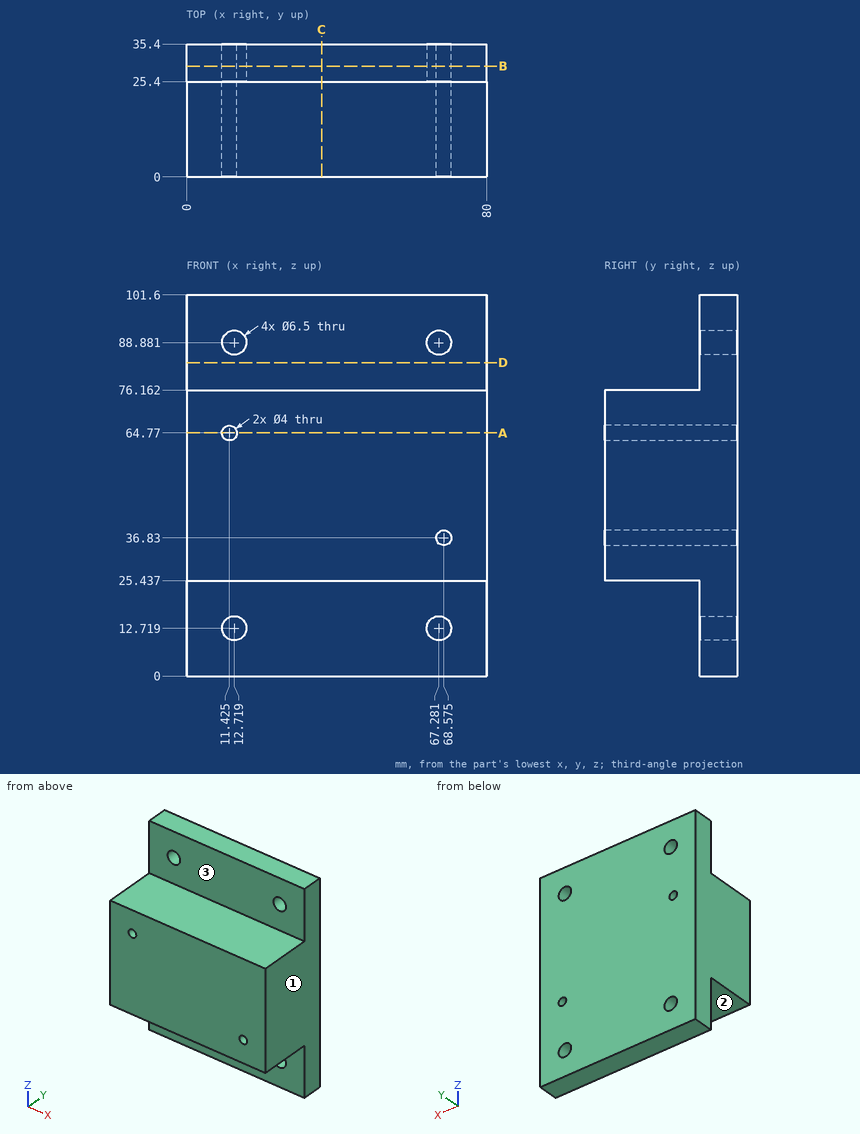
Geometry: see drawing. Coordinates: mm, zero at the bounding-box minimum. A direction names the side the tool comes from. Round coordinates to 2 decimals unless told otherwise and drop trailing zeros. Loops run counter-clockwise (first coordinate to the right, second up) from the corner with the lowest first, then second, coordinate; pieces in that order, holes last. Notation, with made-up numbers: (67.5, 34.25) -> (79.5, 34.25) arc R20 ccw to (79.5, 45.25) -> close; hole circle Ø10 at (-1.5, 35.25). An arc over 180 degrees is marked (long way). Use one line per item in the form item = value. Start each with the question number.
Item 1: Section query D-D on z = 83.5. Return the cut outline in (x, y).
Item 2: Section query A-A on z = 64.77. Return the cut outline in (x, y) (1 decimal), then the cut area to 3 significant figures.
Item 3: Contact query for flat-ended pins moving along their axis: pin 1 Ø4 at (x, z) = (67.28, 12.72) entering from +Y; pin 2 Ø20.5 at (x, y) = (45.5, 8) entering from +Z; pin 3 Ø4 at (x, y) = (35, 14) entering from -Z; pin 4 Ø4 at (x, z) = (70, 13) entering from -Y. Output: stop coordinate, or through.
Item 4: Section query C-C on x = 36. Return the cut outline in (y, z), then the cut area to 3 significant figures.
Item 5: Material intervals for L1, parallel to X at y = 27, z = 64.77 (1 decimal); L2, parallel to Z at x = 47, y = 13; L3, parallel to Y at x = 70.5, z = 92.5, sorted ascending. Write a range as from..to.
Item 6: Set-up query: the marked faces 1, 2 and 3. Return all of +Z, -Z, +X, -X, +Y, -Y with unobstructed straight access to the full face (end or side cutting, diameter ignored); none if empty.
Item 7: Section query B-B on y = 29.5. Count the separate pieces of the cut face and the enclosed holes in it, then the cut area to 3 significant figures.
Ans:
q1.outline = (0, 25.4) -> (80, 25.4) -> (80, 35.4) -> (0, 35.4) -> close
q2.outline = (0, 0) -> (9.4, 0) -> (9.4, 35.4) -> (0, 35.4) -> close; (13.4, 0) -> (80, 0) -> (80, 35.4) -> (13.4, 35.4) -> close
q2.area = 2,690 mm^2
q3.pin_1 = through
q3.pin_2 = 76.16
q3.pin_3 = 25.44
q3.pin_4 = 25.4
q4.outline = (0, 25.44) -> (25.4, 25.44) -> (25.4, 0) -> (35.4, 0) -> (35.4, 101.6) -> (25.4, 101.6) -> (25.4, 76.16) -> (0, 76.16) -> close
q4.area = 2,300 mm^2
q5.L1 = 0..9.4, 13.4..80
q5.L2 = 25.44..76.16
q5.L3 = 25.4..35.4
q6.face_1 = +Z, -Z, +X, +Y, -Y
q6.face_2 = -Z, +X, -X, -Y
q6.face_3 = +Z, +X, -X, -Y
q7.separate_pieces = 1
q7.enclosed_holes = 6
q7.area = 7,970 mm^2
